Model file for the job. Use its own axes, mm. Coordinates: 2 decimals unless noted, no trailing zeros. Write each loop counter-clockwise with the first axis right and the second up, starting at its lowest first coordinate (ties: lowest second). Pieces come first, ordered by that corner, then holes. Notation, with made-up numbers: M -25,62 L 5,62 A21 ccw 5,98 Z; hole C 48.25,13.25 d5. An arc over 180 degrees is marked long. Use CSV: the item, a comma, the result in double quotes. Start each with the question number.
from build123d import *

# Parameters (mm, degrees)
SALIENTE_EXTRUIR1_DEPTH                      = 3.17
CORTAR_EXTRUIR1_REACH                        = 182
CORTAR_EXTRUIR7_START                        = -117.08
CORTAR_EXTRUIR7_DEPTH                        = 117.08
CROQUIS3_R                                   = 1.585
CORTAR_EXTRUIR2_DEPTH                        = 3.17
CORTAR_EXTRUIR3_REACH                        = 5.17
CROQUIS4_R                                   = 1.585
CORTAR_EXTRUIR4_REACH                        = 5.17
CROQUIS6_R                                   = 1.585
CROQUIS7_R                                   = 1.585
CORTAR_EXTRUIR5_DEPTH                        = 3.17
CROQUIS15_R                                  = 4
CORTAR_EXTRUIR6_DEPTH                        = 2
CORTAR_EXTRUIR6_TAPER                        = 50.5
AVELLANADO_PARA_TORNILLO_CON_CABEZA_2_COUNT  = 2
AVELLANADO_PARA_TORNILLO_CON_CABEZA_2_PITCH  = 63.24912037
AVELLANADO_PARA_TORNILLO_CON_CABEZA_3_COUNT  = 2
AVELLANADO_PARA_TORNILLO_CON_CABEZA_3_PITCH  = 83.591620659
AVELLANADO_PARA_TORNILLO_CON_CABEZA_4_COUNT  = 2
AVELLANADO_PARA_TORNILLO_CON_CABEZA_4_PITCH  = 95.923454089
AVELLANADO_PARA_TORNILLO_CON_CABEZA_5_COUNT  = 2
AVELLANADO_PARA_TORNILLO_CON_CABEZA_5_PITCH  = 84.359061325
AVELLANADO_PARA_TORNILLO_CON_CABEZA_6_COUNT  = 2
AVELLANADO_PARA_TORNILLO_CON_CABEZA_6_PITCH  = 108.187112114
AVELLANADO_PARA_TORNILLO_CON_CABEZA_7_COUNT  = 2
AVELLANADO_PARA_TORNILLO_CON_CABEZA_7_PITCH  = 122.968731979
AVELLANADO_PARA_TORNILLO_CON_CABEZA_8_COUNT  = 2
AVELLANADO_PARA_TORNILLO_CON_CABEZA_8_PITCH  = 145.077768953
AVELLANADO_PARA_TORNILLO_CON_CABEZA_9_COUNT  = 2
AVELLANADO_PARA_TORNILLO_CON_CABEZA_9_PITCH  = 143.959894511
AVELLANADO_PARA_TORNILLO_CON_CABEZA_10_COUNT = 2
AVELLANADO_PARA_TORNILLO_CON_CABEZA_10_PITCH = 148


with BuildPart() as part:
    # Croquis1 → Saliente-Extruir1 (new body)
    with BuildSketch(Plane(origin=(0, 0, 0), x_dir=(1, 0, 0), z_dir=(0, 1, 0))):
        Polygon((-62.5, 90), (-62.5, 27.08), (-90, 27.08), (-90, -90), (90, -90), (90, 27.08), (62.5, 27.08), (62.5, 90), align=None)
    extrude(amount=SALIENTE_EXTRUIR1_DEPTH)

    # Croquis2 → Cortar-Extruir1 (cut, up to next)
    with BuildSketch(Plane.ZY.offset(90), mode=Mode.PRIVATE) as cortar_extruir1_sk1:
        Polygon((90, 0), (84.50939894, 3.17), (90, 3.17), align=None)
    cortar_extruir1_tool1 = extrude(cortar_extruir1_sk1.sketch, amount=-CORTAR_EXTRUIR1_REACH, mode=Mode.PRIVATE) & part.part
    add(cortar_extruir1_tool1.solids().sort_by_distance((-90, 2.113333, 88.1698))[0], mode=Mode.SUBTRACT)

    # Croquis16 → Cortar-Extruir7 (cut)
    with BuildSketch(Plane(origin=(0, 0, -27.08), x_dir=(-1, 0, 0), z_dir=(0, 0, -1)).offset(CORTAR_EXTRUIR7_START)):
        Polygon((90, 3.17), (90, 0), (87.780342104, 3.17), align=None)
    cortar_extruir7 = extrude(amount=CORTAR_EXTRUIR7_DEPTH, mode=Mode.SUBTRACT)

    # Simetría4: Cortar-Extruir7 across plane
    add(cortar_extruir7.mirror(Plane(origin=(0, 0, 0), x_dir=(0, 0, 1), z_dir=(1, 0, 0))), mode=Mode.SUBTRACT)

    # Croquis3 → Cortar-Extruir2 (cut)
    with BuildSketch(Plane(origin=(0, 3.17, 0), x_dir=(1, 0, 0), z_dir=(0, 1, 0))):
        with Locations((74, -24.279339937)):
            Circle(CROQUIS3_R)
    cortar_extruir2 = extrude(amount=-CORTAR_EXTRUIR2_DEPTH, mode=Mode.SUBTRACT)

    # Simetría1: Cortar-Extruir2 across plane
    add(cortar_extruir2.mirror(Plane(origin=(0, 0, 0), x_dir=(0, 0, 1), z_dir=(1, 0, 0))), mode=Mode.SUBTRACT)

    # Croquis4 → Cortar-Extruir3 (cut, up to next)
    with BuildSketch(Plane(origin=(0, 3.17, 0), x_dir=(1, 0, 0), z_dir=(0, 1, 0)), mode=Mode.PRIVATE) as cortar_extruir3_sk1:
        with Locations((-56.5, 36.50060106)):
            Circle(CROQUIS4_R)
    cortar_extruir3_tool1 = extrude(cortar_extruir3_sk1.sketch, amount=-CORTAR_EXTRUIR3_REACH, mode=Mode.PRIVATE) & part.part
    add(cortar_extruir3_tool1.solids().sort_by_distance((-56.5, 3.17, -36.500601))[0], mode=Mode.SUBTRACT)
    # Croquis4 → Cortar-Extruir3 (cut, up to next)
    with BuildSketch(Plane(origin=(0, 3.17, 0), x_dir=(1, 0, 0), z_dir=(0, 1, 0)), mode=Mode.PRIVATE) as cortar_extruir3_sk2:
        with Locations((-15.5, 36.50060106)):
            Circle(CROQUIS4_R)
    cortar_extruir3_tool2 = extrude(cortar_extruir3_sk2.sketch, amount=-CORTAR_EXTRUIR3_REACH, mode=Mode.PRIVATE) & part.part
    add(cortar_extruir3_tool2.solids().sort_by_distance((-15.5, 3.17, -36.500601))[0], mode=Mode.SUBTRACT)
    # Croquis4 → Cortar-Extruir3 (cut, up to next)
    with BuildSketch(Plane(origin=(0, 3.17, 0), x_dir=(1, 0, 0), z_dir=(0, 1, 0)), mode=Mode.PRIVATE) as cortar_extruir3_sk3:
        with Locations((-15.5, 85.00060106)):
            Circle(CROQUIS4_R)
    cortar_extruir3_tool3 = extrude(cortar_extruir3_sk3.sketch, amount=-CORTAR_EXTRUIR3_REACH, mode=Mode.PRIVATE) & part.part
    add(cortar_extruir3_tool3.solids().sort_by_distance((-15.5, 3.17, -85.000601))[0], mode=Mode.SUBTRACT)
    # Croquis4 → Cortar-Extruir3 (cut, up to next)
    with BuildSketch(Plane(origin=(0, 3.17, 0), x_dir=(1, 0, 0), z_dir=(0, 1, 0)), mode=Mode.PRIVATE) as cortar_extruir3_sk4:
        with Locations((-56.5, 85.00060106)):
            Circle(CROQUIS4_R)
    cortar_extruir3_tool4 = extrude(cortar_extruir3_sk4.sketch, amount=-CORTAR_EXTRUIR3_REACH, mode=Mode.PRIVATE) & part.part
    add(cortar_extruir3_tool4.solids().sort_by_distance((-56.5, 3.17, -85.000601))[0], mode=Mode.SUBTRACT)

    # Croquis6 → Cortar-Extruir4 (cut, up to next)
    with BuildSketch(Plane(origin=(0, 3.17, 0), x_dir=(1, 0, 0), z_dir=(0, 1, 0)), mode=Mode.PRIVATE) as cortar_extruir4_sk1:
        with Locations((56.5, 85.00060106)):
            Circle(CROQUIS6_R)
    cortar_extruir4_tool1 = extrude(cortar_extruir4_sk1.sketch, amount=-CORTAR_EXTRUIR4_REACH, mode=Mode.PRIVATE) & part.part
    add(cortar_extruir4_tool1.solids().sort_by_distance((56.5, 3.17, -85.000601))[0], mode=Mode.SUBTRACT)
    # Croquis6 → Cortar-Extruir4 (cut, up to next)
    with BuildSketch(Plane(origin=(0, 3.17, 0), x_dir=(1, 0, 0), z_dir=(0, 1, 0)), mode=Mode.PRIVATE) as cortar_extruir4_sk2:
        with Locations((15.5, 85.00060106)):
            Circle(CROQUIS6_R)
    cortar_extruir4_tool2 = extrude(cortar_extruir4_sk2.sketch, amount=-CORTAR_EXTRUIR4_REACH, mode=Mode.PRIVATE) & part.part
    add(cortar_extruir4_tool2.solids().sort_by_distance((15.5, 3.17, -85.000601))[0], mode=Mode.SUBTRACT)
    # Croquis6 → Cortar-Extruir4 (cut, up to next)
    with BuildSketch(Plane(origin=(0, 3.17, 0), x_dir=(1, 0, 0), z_dir=(0, 1, 0)), mode=Mode.PRIVATE) as cortar_extruir4_sk3:
        with Locations((15.5, 36.50060106)):
            Circle(CROQUIS6_R)
    cortar_extruir4_tool3 = extrude(cortar_extruir4_sk3.sketch, amount=-CORTAR_EXTRUIR4_REACH, mode=Mode.PRIVATE) & part.part
    add(cortar_extruir4_tool3.solids().sort_by_distance((15.5, 3.17, -36.500601))[0], mode=Mode.SUBTRACT)
    # Croquis6 → Cortar-Extruir4 (cut, up to next)
    with BuildSketch(Plane(origin=(0, 3.17, 0), x_dir=(1, 0, 0), z_dir=(0, 1, 0)), mode=Mode.PRIVATE) as cortar_extruir4_sk4:
        with Locations((56.5, 36.50060106)):
            Circle(CROQUIS6_R)
    cortar_extruir4_tool4 = extrude(cortar_extruir4_sk4.sketch, amount=-CORTAR_EXTRUIR4_REACH, mode=Mode.PRIVATE) & part.part
    add(cortar_extruir4_tool4.solids().sort_by_distance((56.5, 3.17, -36.500601))[0], mode=Mode.SUBTRACT)

    # Croquis7 → Cortar-Extruir5 (cut)
    with BuildSketch(Plane(origin=(0, 3.17, 0), x_dir=(1, 0, 0), z_dir=(0, 1, 0))):
        with Locations((-20, 85.00060106)):
            Circle(CROQUIS7_R)
        with Locations((-47.5, 85.00060106)):
            Circle(CROQUIS7_R)
        with Locations((-47.5, 55.00060106)):
            Circle(CROQUIS7_R)
        with Locations((-20, 55.00060106)):
            Circle(CROQUIS7_R)
    cortar_extruir5 = extrude(amount=-CORTAR_EXTRUIR5_DEPTH, mode=Mode.SUBTRACT)

    # Simetría2: Cortar-Extruir5 across plane
    add(cortar_extruir5.mirror(Plane(origin=(0, 0, 0), x_dir=(0, 0, 1), z_dir=(1, 0, 0))), mode=Mode.SUBTRACT)

    # Croquis15 → Cortar-Extruir6 (cut)
    with BuildSketch(Plane(origin=(0, 0, 0), x_dir=(-1, 0, 0), z_dir=(0, -1, 0))):
        with Locations((20, 55.00060106)):
            Circle(CROQUIS15_R)
        with Locations((15.5, 36.50060106)):
            Circle(CROQUIS15_R)
        with Locations((56.5, 36.50060106)):
            Circle(CROQUIS15_R)
        with Locations((47.5, 55.00060106)):
            Circle(CROQUIS15_R)
        with Locations((56.5, 85.00060106)):
            Circle(CROQUIS15_R)
        with Locations((47.5, 85.00060106)):
            Circle(CROQUIS15_R)
        with Locations((74, -24.279339937)):
            Circle(CROQUIS15_R)
    cortar_extruir6 = extrude(amount=-CORTAR_EXTRUIR6_DEPTH, taper=CORTAR_EXTRUIR6_TAPER, mode=Mode.SUBTRACT)

    # Simetría3: Cortar-Extruir6 across plane
    add(cortar_extruir6.mirror(Plane(origin=(0, 0, 0), x_dir=(0, 0, 1), z_dir=(1, 0, 0))), mode=Mode.SUBTRACT)

    # Croquis14 → Avellanado para tornillo con cabeza avellanada en cruz de M3.51 (revolve, cut)
    with BuildSketch(Plane(origin=(74, 0, 24.279339937), x_dir=(0, 0, -1), z_dir=(1, 0, 0))):
        Polygon((0, 0), (0, 3.17), (1.95, 3.17), (1.95, 1.979661988), (4, 0), align=None)
    avellanado_para_tornillo_con_cabeza_avel = revolve(axis=Axis((74, -6.35, 24.279339937), (0, 1, 0)), mode=Mode.SUBTRACT)

    # Avellanado para tornillo con cabeza  2: Avellanado para tornillo con cabeza avellanada en cruz de M3.51 ×2
    with Locations(*[Vector(-0.27668369, 0, -0.960961048) * (i * AVELLANADO_PARA_TORNILLO_CON_CABEZA_2_PITCH) for i in range(1, AVELLANADO_PARA_TORNILLO_CON_CABEZA_2_COUNT)]):
        add(avellanado_para_tornillo_con_cabeza_avel, mode=Mode.SUBTRACT)

    # Avellanado para tornillo con cabeza  3: Avellanado para tornillo con cabeza avellanada en cruz de M3.51 ×2
    with Locations(*[Vector(-0.317017421, 0, -0.948419714) * (i * AVELLANADO_PARA_TORNILLO_CON_CABEZA_3_PITCH) for i in range(1, AVELLANADO_PARA_TORNILLO_CON_CABEZA_3_COUNT)]):
        add(avellanado_para_tornillo_con_cabeza_avel, mode=Mode.SUBTRACT)

    # Avellanado para tornillo con cabeza  4: Avellanado para tornillo con cabeza avellanada en cruz de M3.51 ×2
    with Locations(*[Vector(-0.562948869, 0, -0.826491725) * (i * AVELLANADO_PARA_TORNILLO_CON_CABEZA_4_PITCH) for i in range(1, AVELLANADO_PARA_TORNILLO_CON_CABEZA_4_COUNT)]):
        add(avellanado_para_tornillo_con_cabeza_avel, mode=Mode.SUBTRACT)

    # Avellanado para tornillo con cabeza  5: Avellanado para tornillo con cabeza avellanada en cruz de M3.51 ×2
    with Locations(*[Vector(-0.693464331, 0, -0.720490959) * (i * AVELLANADO_PARA_TORNILLO_CON_CABEZA_5_PITCH) for i in range(1, AVELLANADO_PARA_TORNILLO_CON_CABEZA_5_COUNT)]):
        add(avellanado_para_tornillo_con_cabeza_avel, mode=Mode.SUBTRACT)

    # Avellanado para tornillo con cabeza  6: Avellanado para tornillo con cabeza avellanada en cruz de M3.51 ×2
    with Locations(*[Vector(-0.827270441, 0, -0.561803895) * (i * AVELLANADO_PARA_TORNILLO_CON_CABEZA_6_PITCH) for i in range(1, AVELLANADO_PARA_TORNILLO_CON_CABEZA_6_COUNT)]):
        add(avellanado_para_tornillo_con_cabeza_avel, mode=Mode.SUBTRACT)

    # Avellanado para tornillo con cabeza  7: Avellanado para tornillo con cabeza avellanada en cruz de M3.51 ×2
    with Locations(*[Vector(-0.764421967, 0, -0.64471626) * (i * AVELLANADO_PARA_TORNILLO_CON_CABEZA_7_PITCH) for i in range(1, AVELLANADO_PARA_TORNILLO_CON_CABEZA_7_COUNT)]):
        add(avellanado_para_tornillo_con_cabeza_avel, mode=Mode.SUBTRACT)

    # Avellanado para tornillo con cabeza  8: Avellanado para tornillo con cabeza avellanada en cruz de M3.51 ×2
    with Locations(*[Vector(-0.837481861, 0, -0.546465124) * (i * AVELLANADO_PARA_TORNILLO_CON_CABEZA_8_PITCH) for i in range(1, AVELLANADO_PARA_TORNILLO_CON_CABEZA_8_COUNT)]):
        add(avellanado_para_tornillo_con_cabeza_avel, mode=Mode.SUBTRACT)

    # Avellanado para tornillo con cabeza  9: Avellanado para tornillo con cabeza avellanada en cruz de M3.51 ×2
    with Locations(*[Vector(-0.90650247, 0, -0.422200511) * (i * AVELLANADO_PARA_TORNILLO_CON_CABEZA_9_PITCH) for i in range(1, AVELLANADO_PARA_TORNILLO_CON_CABEZA_9_COUNT)]):
        add(avellanado_para_tornillo_con_cabeza_avel, mode=Mode.SUBTRACT)

    # Avellanado para tornillo con cabeza  10: Avellanado para tornillo con cabeza avellanada en cruz de M3.51 ×2
    with Locations(*[(-i * AVELLANADO_PARA_TORNILLO_CON_CABEZA_10_PITCH, 0, 0) for i in range(1, AVELLANADO_PARA_TORNILLO_CON_CABEZA_10_COUNT)]):
        add(avellanado_para_tornillo_con_cabeza_avel, mode=Mode.SUBTRACT)


solid = part.part
1) Band-saw the part on A-A on y = 0.65. State how many separate pieces and enclosed holes the cut face has, then the cut area to 3 significant figures.
2) Band-saw the part on B-B on x = 8.5. List the corners of the cut face in (y, z).
3) Drop flat-ended pins along their axis: P1, Ø2.5, axis at x = -56.5, z = -85, coming from the -Y side; P2, Ø6, axis at x = 15.5, z = -36.5, coming from the -Y side; P3, Ø1, axis at y = 3, z = 24, coming from the +X side; P4, Ø1.6, axis at x = 75.5, y = 2.5, coming from the -Z side. Give the stop position or say it passes through.
4) Two-plate mould, pull along Z, no slides. Class faces 1 (the face through (72.067, 2.566, 24.533)), 2 (the face through (-1.26, 1.563, 87.293)), 3 (the face through (-1, 3.17, -4)), 4 (the face through (46.88, 1.86, -56.98)): pulls with the +Z half, pulls with the -Z half, needs draft (parallel to the pull), parting line crosses it, or undercut.
5) Wall check: L1, parallel to X at y = 1.2, z = -34.5; L2, parallel to Z at x = -17.5, y = 0.55; L3, parallel to Z at x = 57, y = 0.9. Give the ranges that are in metal, low to high. Write a range as [from, to].
Findings below:
1,separate pieces,"1"
1,enclosed holes,"18"
1,area,"28,100 mm2"
2,outline,"M 0,-90 L 3.17,-90 L 3.17,84.51 L 0,90 Z"
3,P1,"passes through"
3,P2,"stops at y = 0.97"
3,P3,"stops at x = 88.25"
3,P4,"stops at z = -27.08"
4,face 1,"undercut"
4,face 2,"pulls with the +Z half"
4,face 3,"needs draft"
4,face 4,"undercut"
5,L1,"x = [-62.5, -58.4], [-54.6, -17.4], [-13.6, 13.6], [17.4, 54.6], [58.4, 62.5]"
5,L2,"z = [-90, -57.35], [-52.65, -39.29], [-33.71, 89.05]"
5,L3,"z = [-90, -87.87], [-82.14, -39.53], [-33.47, 88.44]"
